Here's how the part is built. I have some questions about the finished solid (model axes, mm). Face numbers are marked on the shaded views. Give positions to 0.01 mm unless a question says otherwise; leave off trailing zeros. Order: outer loops, then holes, each group sorted by start corner. A loop starts at its lowest first (then second) coordinate and runs counter-clockwise, first axis right, second up. Notation, with made-up numbers: (51, 57.25) - (110, 57.25) arc R5 ccw to (110, 61.25) - close; hole circle Ø4 at (77.5, -35). An arc over 180 degrees is marked (long way). One line per question, with ' | ' between items.
from build123d import *

# Parameters (mm, degrees)
EXTRUDE_1_DEPTH     = 10
SKETCH_2_W          = 50
SKETCH_2_H          = 50
CUT_EXTRUDE_1_DEPTH = 3
SKETCH_3_R          = 1.5
CUT_EXTRUDE_2_DEPTH = 87


with BuildPart() as part:
    # 草图1 → 凸台-拉伸1 (new body)
    with BuildSketch(Plane.XY):
        with BuildLine():
            Line((-40, -43), (40, -43))
            ThreePointArc((40, -43), (42.121320344, -42.121320344), (43, -40))
            Line((43, -40), (43, 40))
            ThreePointArc((43, 40), (42.121320344, 42.121320344), (40, 43))
            Line((40, 43), (-40, 43))
            ThreePointArc((-40, 43), (-42.121320344, 42.121320344), (-43, 40))
            Line((-43, 40), (-43, -40))
            ThreePointArc((-43, -40), (-42.121320344, -42.121320344), (-40, -43))
        make_face()
    extrude(amount=EXTRUDE_1_DEPTH)

    # 草图2 → 切除-拉伸1 (cut)
    with BuildSketch(Plane.XY.offset(10)):
        Rectangle(SKETCH_2_W, SKETCH_2_H)
    extrude(amount=-CUT_EXTRUDE_1_DEPTH, mode=Mode.SUBTRACT)

    # 草图3 → 切除-拉伸2 (cut, symmetric)
    with BuildSketch(Plane.XY.offset(10)):
        with Locations((-35, -35)):
            Circle(SKETCH_3_R)
        with Locations((-35, 35)):
            Circle(SKETCH_3_R)
        with Locations((35, -35)):
            Circle(SKETCH_3_R)
        with Locations((35, 35)):
            Circle(SKETCH_3_R)
    extrude(amount=CUT_EXTRUDE_2_DEPTH, both=True, mode=Mode.SUBTRACT)


solid = part.part
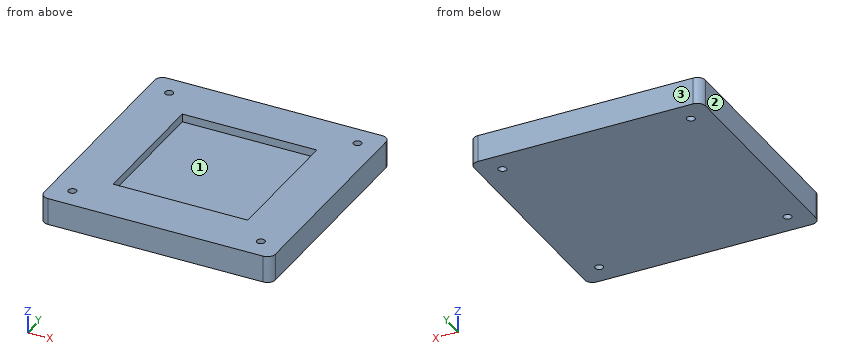
1) I want a section at A-A (x = -35). List the corners of the cut face in (y, z) for me, plus the area to 3 significant figures.
Model answer:
outline: (-43, 0) - (-36.5, 0) - (-36.5, 10) - (-43, 10) - close; (-33.5, 0) - (33.5, 0) - (33.5, 10) - (-33.5, 10) - close; (36.5, 0) - (43, 0) - (43, 10) - (36.5, 10) - close | area: 800 mm2
2) Please list where these lines run through material, in increasing order: L1, parallel to Y at x = -35, z = 4.25; L2, parallel to X at y = 15.5, z = 7.25.
Model answer:
L1: y = -43 to -36.5, -33.5 to 33.5, 36.5 to 43 | L2: x = -43 to -25, 25 to 43
3) I want a section at C-C (z = 8.5). List the corners of the cut face in (x, y) for me.
Model answer:
outline: (-43, -40) arc R3 ccw to (-40, -43) - (40, -43) arc R3 ccw to (43, -40) - (43, 40) arc R3 ccw to (40, 43) - (-40, 43) arc R3 ccw to (-43, 40) - close; hole circle Ø3 at (-35, -35); hole circle Ø3 at (-35, 35); hole (-25, -25) - (25, -25) - (25, 25) - (-25, 25) - close; hole circle Ø3 at (35, -35); hole circle Ø3 at (35, 35)
4) I'm going to push a flat-ended pin straight in: P1, Ø15, axis at x = -9, y = -11, coming from the +Z side. Where does the tip first touch, or does it pass through?
Model answer:
P1: stops at z = 7
5) I want a section at D-D (y = -4.5). List the corners of the cut face in (x, z) for me, plus the area to 3 significant figures.
Model answer:
outline: (-43, 0) - (43, 0) - (43, 10) - (25, 10) - (25, 7) - (-25, 7) - (-25, 10) - (-43, 10) - close | area: 710 mm2
6) Thinking about a two-plate mould opening in Y: for the marked faces 1, 2 and 3, which applies, +Y half, -Y half, draft (parallel to the pull), parting line (faces both ways), or undercut?
Model answer:
face 1: undercut | face 2: draft | face 3: +Y half
